```python
from build123d import *

# Parameters (mm, degrees)
SKETCH1_W           = 35
SKETCH1_H           = 29
BOSS_EXTRUDE1_DEPTH = 57
SKETCH3_W           = 31
SKETCH3_H           = 29
CUT_EXTRUDE1_DEPTH  = 55
FILLET1_R           = 1
CHAMFER1_SIZE       = 2.5
SKETCH4_R           = 1.25
CUT_EXTRUDE2_DEPTH  = 40.5
SKETCH7_R           = 1.25
CUT_EXTRUDE3_DEPTH  = 5


with BuildPart() as part:
    # Sketch1 → Boss-Extrude1 (new body)
    with BuildSketch(Plane.XY):
        with Locations((17.5, 14.5)):
            Rectangle(SKETCH1_W, SKETCH1_H)
    extrude(amount=BOSS_EXTRUDE1_DEPTH)

    # Sketch3 → Cut-Extrude1 (cut)
    with BuildSketch(Plane.XY.offset(57)):
        with Locations((17.5, 14.5)):
            Rectangle(SKETCH3_W, SKETCH3_H)
    extrude(amount=-CUT_EXTRUDE1_DEPTH, mode=Mode.SUBTRACT)

    # Fillet1
    fillet1_edges = [part.edges().sort_by_distance(p)[0] for p in [
        (0, 14.5, 0),
        (35, 14.5, 0),
    ]]
    fillet(fillet1_edges, radius=FILLET1_R)

    # Chamfer1
    chamfer1_edges = [part.edges().sort_by_distance(p)[0] for p in [
        (1, 0, 57),
        (1, 29, 57),
        (34, 0, 57),
        (34, 29, 57),
    ]]
    chamfer(chamfer1_edges, length=CHAMFER1_SIZE)

    # Sketch4 → Cut-Extrude2 (cut)
    with BuildSketch(Plane.ZY):
        with Locations((54.5, 22.5)):
            Circle(SKETCH4_R)
        with Locations((54.5, 6.5)):
            Circle(SKETCH4_R)
    extrude(amount=-CUT_EXTRUDE2_DEPTH, mode=Mode.SUBTRACT)

    # Sketch7 → Cut-Extrude3 (cut)
    with BuildSketch(Plane.XY.offset(2)):
        with Locations((9.5, 6.5)):
            Circle(SKETCH7_R)
        with Locations((17.5, 6.5)):
            Circle(SKETCH7_R)
        with Locations((25.5, 6.5)):
            Circle(SKETCH7_R)
        with Locations((25.5, 14.5)):
            Circle(SKETCH7_R)
        with Locations((17.5, 22.5)):
            Circle(SKETCH7_R)
        with Locations((25.5, 22.5)):
            Circle(SKETCH7_R)
        with Locations((9.5, 14.5)):
            Circle(SKETCH7_R)
        with Locations((9.5, 22.5)):
            Circle(SKETCH7_R)
    extrude(amount=-CUT_EXTRUDE3_DEPTH, mode=Mode.SUBTRACT)


solid = part.part
```
Geometry check sheet. Reference: the model listing, model coordinates, mm. A direction names the side the tool comes from. Coordinates: 2 decimals unless noted, no trailing zeros. Order: outer loops, then holes, each group sorted by start corner. A loop starts at its lowest first (then second) coordinate and runs counter-clockwise, first axis right, second up. Notation, with made-up numbers: (80.5, -4.75) - (120.5, -4.75) arc R22 cw to (120.5, 22.25) - close; hole circle Ø4 at (38.5, 4.25). An arc over 180 degrees is marked (long way). Answer in a Markdown table with one row per item. Add a question column.
1. Gauge pin test, flat end, axial feed: pin 1 Ø3 at (x, y) = (9.5, 6.5) entering from +Z. Record the tip position at first contact, or that the pin passes through.
2. Section check A-A (x = 17.5). Enter the section's corners in (y, z), plus the area to 3 significant figures.
3. Draft check along X on faces 1 (the face through (26.655, 22.021, 1.014)), 2 (the face through (33.99, 6.88, 55.69)), 3 (the face through (8.51, 5.74, 1.01)). Enter one of: +X half, -X half, draft (parallel to the pull), parting line (faces both ways), or undercut.
4. Material ranges on L1, parallel to Y at x = 0.5, z = 54.5; L2, parallel to Y at x = 9.5, z = 1.35; L3, parallel to X at y = 6.5, z = 32, recorded low to high. Write a range as [from, to].
5. Section check B-B (z = 47). Enter the section's corners in (x, y), plus the area to 3 significant figures.
6. Access from +Z, -Z, +X, -X, +Y, -Y to the whole of each face (thin tool, end or side, straight path). Record for faces 4 (the face through (2, 14, 30)), 5 (the face through (0.99, 6.88, 55.69)).
7. Section check D-D (y = 22.5). Give the number of separate pieces and of enclosed holes in the cut face, plus the area to 3 significant figures.
8. Section check C-C (x = 9.5). Enter the section's corners in (y, z).
Data:
| question | item | result |
|---|---|---|
| 1 | pin 1 | stops at z = 2 |
| 2 | outline | (0, 0) - (5.25, 0) - (5.25, 2) - (0, 2) - close; (7.75, 0) - (21.25, 0) - (21.25, 2) - (7.75, 2) - close; (23.75, 0) - (29, 0) - (29, 2) - (23.75, 2) - close |
| 2 | area | 48.0 mm² |
| 3 | face 1 | undercut |
| 3 | face 2 | draft |
| 3 | face 3 | undercut |
| 4 | L1 | y = [0, 5.25], [7.75, 21.25], [23.75, 29] |
| 4 | L2 | y = [0, 5.25], [7.75, 13.25], [15.75, 21.25], [23.75, 29] |
| 4 | L3 | x = [0, 2], [33, 35] |
| 5 | outline | (0, 0) - (2, 0) - (2, 29) - (0, 29) - close; (33, 0) - (35, 0) - (35, 29) - (33, 29) - close |
| 5 | area | 116 mm² |
| 6 | face 4 | +Z, +Y, -Y |
| 6 | face 5 | +X, -X |
| 7 | separate pieces | 6 |
| 7 | enclosed holes | 0 |
| 7 | area | 265 mm² |
| 8 | outline | (0, 0) - (5.25, 0) - (5.25, 2) - (0, 2) - close; (7.75, 0) - (13.25, 0) - (13.25, 2) - (7.75, 2) - close; (15.75, 0) - (21.25, 0) - (21.25, 2) - (15.75, 2) - close; (23.75, 0) - (29, 0) - (29, 2) - (23.75, 2) - close |
